```python
from build123d import *

# Parameters (mm, degrees)
SKETCH_1_W          = 100
SKETCH_1_H          = 100
EXTRUDE_1_DEPTH     = 10
CUT_EXTRUDE_3_DEPTH = 27
CUT_EXTRUDE_4_DEPTH = 27
SKETCH_5_R          = 1.6
CUT_EXTRUDE_5_DEPTH = 27
SKETCH_6_W          = 37
SKETCH_6_H          = 5
SKETCH_6_W_2        = 7.5
CUT_EXTRUDE_6_DEPTH = 27
SKETCH_8_W          = 3.805881933
SKETCH_8_H          = 5
EXTRUDE_2_DEPTH     = 7
SKETCH_10_W         = 3.75
SKETCH_10_H         = 5
EXTRUDE_3_DEPTH     = 7
FILLET_1_R          = 5
FILLET_2_R          = 5
SKETCH_14_W         = 7
SKETCH_14_H         = 5
EXTRUDE_6_DEPTH     = 3.750003
CUT_EXTRUDE_START   = -3.805882
CUT_EXTRUDE_8_DEPTH = 3.805882


with BuildPart() as part:
    # 草图1 → 凸台-拉伸1 (new body)
    with BuildSketch(Plane(origin=(0, 0, 0), x_dir=(1, 0, 0), z_dir=(0, 1, 0))):
        with Locations((50, -50)):
            Rectangle(SKETCH_1_W, SKETCH_1_H)
    extrude(amount=EXTRUDE_1_DEPTH)

    # 草图2 → 切除-拉伸3 (cut)
    with BuildSketch(Plane(origin=(0, 10, 0), x_dir=(1, 0, 0), z_dir=(0, 1, 0))):
        Polygon((50.15455276, -13), (20.65455276, -13), (0, -13), (0, -100), (100, -100), (100, -13), align=None)
    extrude(amount=-CUT_EXTRUDE_3_DEPTH, mode=Mode.SUBTRACT)

    # 草图4 → 切除-拉伸4 (cut)
    with BuildSketch(Plane(origin=(0, 10, 0), x_dir=(1, 0, 0), z_dir=(0, 1, 0))):
        Polygon((13.15455276, -13), (13.15455276, -6.5), (13.15455276, 0), (0, 0), (0, -13), align=None)
        Polygon((100, 0), (57.65455276, 0), (57.65455276, -6.5), (57.65455276, -13), (100, -13), align=None)
    extrude(amount=-CUT_EXTRUDE_4_DEPTH, mode=Mode.SUBTRACT)

    # 草图5 → 切除-拉伸5 (cut)
    with BuildSketch(Plane(origin=(0, 10, 0), x_dir=(1, 0, 0), z_dir=(0, 1, 0))):
        with Locations(Location((16.90455276, -6.5, 0), (0, 0, 270))):
            Circle(SKETCH_5_R)
        with Locations(Location((53.90455276, -6.5, 0), (0, 0, 270))):
            Circle(SKETCH_5_R)
    extrude(amount=-CUT_EXTRUDE_5_DEPTH, mode=Mode.SUBTRACT)

    # 草图6 → 切除-拉伸6 (cut)
    with BuildSketch(Plane.XY.offset(13)):
        with Locations((31.65455276, 2.5)):
            Rectangle(SKETCH_6_W, SKETCH_6_H)
        with Locations((53.90455276, 2.5)):
            Rectangle(SKETCH_6_W_2, SKETCH_6_H)
    extrude(amount=-CUT_EXTRUDE_6_DEPTH, mode=Mode.SUBTRACT)

    # 草图8 → 凸台-拉伸2 (add)
    with BuildSketch(Plane.XY.offset(13)):
        with Locations((55.751611794, 7.5)):
            Rectangle(SKETCH_8_W, SKETCH_8_H)
    extrude(amount=EXTRUDE_2_DEPTH)

    # 草图10 → 凸台-拉伸3 (add)
    with BuildSketch(Plane(origin=(0, 0, 0), x_dir=(-1, 0, 0), z_dir=(0, 0, -1))):
        with Locations((-55.77955276, 7.5)):
            Rectangle(SKETCH_10_W, SKETCH_10_H)
    extrude(amount=EXTRUDE_3_DEPTH)

    # 圆角1
    fillet_1_edges = [part.edges().sort_by_distance(p)[0] for p in [
        (13.15455276, 7.5, 0),
    ]]
    fillet(fillet_1_edges, radius=FILLET_1_R)

    # 圆角2
    fillet_2_edges = [part.edges().sort_by_distance(p)[0] for p in [
        (13.15455276, 7.5, 13),
    ]]
    fillet(fillet_2_edges, radius=FILLET_2_R)

    # 草图14 → 凸台-拉伸6 (add)
    with BuildSketch(Plane(origin=(57.65455276, 0, 0), x_dir=(0, 0, -1), z_dir=(1, 0, 0))):
        with Locations((-16.5, 12.5)):
            Rectangle(SKETCH_14_W, SKETCH_14_H)
        with Locations((-16.5, 2.5)):
            Rectangle(SKETCH_14_W, SKETCH_14_H)
        with Locations((3.5, 12.5)):
            Rectangle(SKETCH_14_W, SKETCH_14_H)
        with Locations((3.5, 2.5)):
            Rectangle(SKETCH_14_W, SKETCH_14_H)
    extrude(amount=-EXTRUDE_6_DEPTH)

    # 草图15 → 切除-拉伸8 (cut)
    with BuildSketch(Plane.ZY.offset(-53.848670827).offset(CUT_EXTRUDE_START)):
        with BuildLine():
            ThreePointArc((-1.9, 7.5), (-1.976327186, 7.98828389), (-2.198026446, 8.42998111))
            Line((-2.198026446, 8.42998111), (-4.801973554, 6.57001889))
            ThreePointArc((-4.801973554, 6.57001889), (-3.01171611, 5.976327186), (-1.9, 7.5))
        make_face()
        with BuildLine():
            Line((-4.801973554, 6.57001889), (-2.198026446, 8.42998111))
            ThreePointArc((-2.198026446, 8.42998111), (-4.42998111, 8.801973554), (-4.801973554, 6.57001889))
        make_face()
        with BuildLine():
            ThreePointArc((18.1, 7.5), (16.98828389, 9.023672814), (15.198026446, 8.42998111))
            Line((15.198026446, 8.42998111), (17.801973554, 6.57001889))
            ThreePointArc((17.801973554, 6.57001889), (18.023672814, 7.01171611), (18.1, 7.5))
        make_face()
        with BuildLine():
            Line((17.801973554, 6.57001889), (15.198026446, 8.42998111))
            ThreePointArc((15.198026446, 8.42998111), (15.57001889, 6.198026446), (17.801973554, 6.57001889))
        make_face()
    extrude(amount=CUT_EXTRUDE_8_DEPTH, mode=Mode.SUBTRACT)


solid = part.part
```
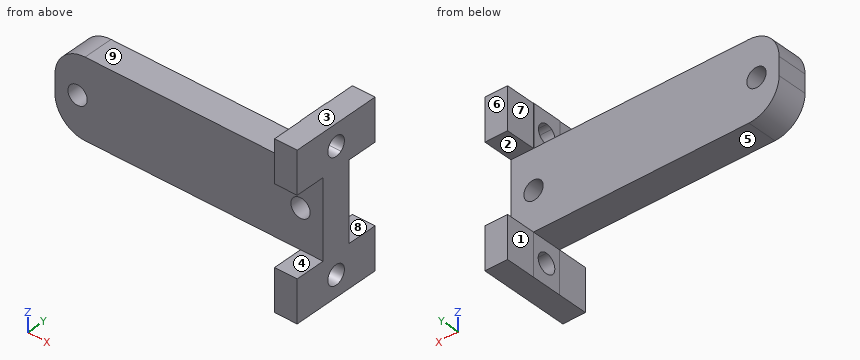
Can you work these out from the model? Positions are in its coordinate system, mm. Face numbers are marked on the shaded views. A direction names the side the tool comes from. Coordinates: 2 decimals unless noted, no trailing zeros. Order: outer loops, then holes, each group sorted by start corner. A loop starts at its lowest first (then second) coordinate and runs counter-clockwise, first axis right, second up.
1. I need wall thicknesses on line 1 (X direction, y = 8.7, z = 6.5); line 2 (Y direction, x = 30, z = 12.75); line 3 (X direction, y = 8.5, z = 14.5). Which ranges of each line are inside material? Lowest first, please.
2. Thinking about a two-plate mould opening in Z: for the marked faces 1, 2, 3 and 4, which applies, +Z half, -Z half, draft (parallel to the pull), parting line (faces both ways), or undercut?
3. If we section it at A-A (z = 16.5): Please give me the cut outline in (x, y).
4. For the marked faces 5, 6, 7, 8 and 9, which set-ups out of +Z, -Z, +X, -X, +Y, -Y let a thin tool reach every point of the face, with its end or its side?
5. If we section it at B-B (y = 3): Please give me the cut outline in (x, z).
6. I'm going to push flat-ended pins straight in: pin 1 (6 mm diameter, centred on x = 27, z = 10.5, fed in from -Y); pin 2 (5.5 mm diameter, centred on y = 13, z = -4, fed in from -X); pin 3 (2.5 mm diameter, centred on x = 43.5, y = 7.5, fed in from +Z). Where does each tip first touch, or does it pass through?
7. If we section it at C-C (z = 6.5): Please give me the cut outline in (x, y).
Entries:
1. line 1: x = 13.15 to 15.3, 18.5 to 52.3, 55.5 to 57.65
1. line 2: y = 5 to 10
1. line 3: x = 53.85 to 57.65
2. face 1: draft
2. face 2: undercut
2. face 3: +Z half
2. face 4: undercut
3. outline: (53.85, 5) - (53.9, 5) - (53.9, 0) - (57.65, 0) - (57.65, 5.9) - (53.85, 5.9) - close; (53.85, 9.1) - (57.65, 9.1) - (57.65, 15) - (53.9, 15) - (53.9, 10) - (53.85, 10) - close
4. face 5: -Z, -X, +Y, -Y
4. face 6: +Z, -Z, +X, -X, +Y
4. face 7: +Z, -Z, -X, +Y
4. face 8: +X, -X, +Y
4. face 9: +Z, -X, +Y, -Y
5. outline: (53.9, -7) - (57.65, -7) - (57.65, 0) - (53.9, 0) - close; (53.9, 13) - (57.65, 13) - (57.65, 20) - (53.9, 20) - close
6. pin 1: stops at y = 5
6. pin 2: stops at x = 53.9
6. pin 3: stops at z = 13
7. outline: (13.15, 5) - (15.3, 5) - (15.3, 10) - (13.15, 10) - close; (18.5, 5) - (52.3, 5) - (52.3, 10) - (18.5, 10) - close; (55.5, 5) - (57.65, 5) - (57.65, 10) - (55.5, 10) - close
